Design review of the part built by this model. Coordinates are the model's own, in mm. A direction names the side the tool comes from. Coordinates: 2 decimals unless noted, no trailing zeros. Write each loop counter-clockwise with the first axis right and the second up, starting at its lowest first coordinate (ties: lowest second). Pieces come first, ordered by that corner, then holes. Notation, with made-up numbers: (62, -3.5) -> (73, -3.5) arc R16 ccw to (73, 2.5) -> close; hole circle Ø8 at (89.5, 29). An arc over 180 degrees is marked (long way). One line per question, with ' | ' between items. Start each with the question number.
Q1. Add section B-B on z = -4. State the section outline as (x, y) points, and give its area (3 significant figures).
Q2. For P1, Ø2, axis at x = 3, z = 1.5, coming from the +Y side; P2, Ø1.8, axis at x = -0.5, y = 0.5, coming from the -Z side (3 decimals); P3, Ø1.5, axis at y = 1, z = 3, coming from the -X side; P4, Ø10, axis at y = 3, z = 7, coming from the +X side, all flat-tipped, find the tip position at first contact; note any pin that passes through.
Q3. Add section A-A on y = 7.5. State the section outline as (x, z) points.
Q4. Add section C-C on y = -6. State the section outline as (x, z) points.
Q5. Add section D-D on x = 0. State the section outline as (y, z) points (3 decimals), and give its area (3 significant figures).
Q6. For faces 1 (the flat face through (0, 0, 12.5)), 2 (the flat face through (-4.762, -1, -11)), 3 (the flat face through (5.08, 7, 0)), list the 3-axis set-ups (+Z, -Z, +X, -X, +Y, -Y) from which the entire face can be reached by the end or side of a thin tool; tool diameter is ignored.
Q7. Wall thickness on probe 1 along Y at (x, z) = (0, -1.25); probe 2 along X at (y, z) = (6, 8.5); probe 3 along X at (y, z) = (5.5, 10): over which ranges is each line inside the solid? List them lowest first.
Q8. Draft analysis for pull direction X (two halves, no side actions). For faces 4 (the cylindrical face through (20.5, -0.13, 11.47)), 5 (the flat face through (4.762, -1, -11)), 6 (the flat face through (11, 9.6, 3)), state which applies: pulls with the +X half, pulls with the -X half, needs draft (parallel to the pull), parting line crosses it, or undercut.
from build123d import *

# Parameters (mm, degrees)
BOSS_EXTRUDE1_DEPTH = 9.6
FILLET5_R           = 2
SKETCH7_W           = 10.16
SKETCH7_H           = 5.28
CUT_EXTRUDE6_DEPTH  = 34.879754173
SKETCH11_W          = 9.525
SKETCH11_H          = 9.525
CUT_EXTRUDE9_DEPTH  = 3.375
SKETCH12_R          = 1.5
CUT_EXTRUDE10_DEPTH = 9.525


with BuildPart() as part:
    # Sketch1 → Boss-Extrude1 (new, symmetric)
    with BuildSketch(Plane(origin=(0, 0, 0), x_dir=(1, 0, 0), z_dir=(0, 1, 0))):
        Polygon((-14.297771125, -12.5), (14.297771125, -12.5), (22.216878365, -12.5), (7.783121635, 12.5), (-7.783121635, 12.5), (-22.216878365, -12.5), align=None)
    extrude(amount=BOSS_EXTRUDE1_DEPTH, both=True)

    # Fillet5
    fillet5_edges = [part.edges().sort_by_distance(p)[0] for p in [
        (-22.216878365, 0, 12.5),
        (-7.783121635, 0, -12.5),
        (7.783121635, 0, -12.5),
        (22.216878365, 0, 12.5),
    ]]
    fillet(fillet5_edges, radius=FILLET5_R)

    # Sketch7 → Cut-Extrude6 (cut, through all)
    with BuildSketch(Plane.XY.offset(12.5)):
        with Locations((0, 6.96)):
            Rectangle(SKETCH7_W, SKETCH7_H)
    extrude(amount=-CUT_EXTRUDE6_DEPTH, mode=Mode.SUBTRACT)

    # Sketch11 → Cut-Extrude9 (cut)
    with BuildSketch(Plane(origin=(0, 0, -12.5), x_dir=(-1, 0, 0), z_dir=(0, 0, -1))):
        with Locations((0, -0.4425)):
            Rectangle(SKETCH11_W, SKETCH11_H)
    extrude(amount=-CUT_EXTRUDE9_DEPTH, mode=Mode.SUBTRACT)

    # Sketch12 → Cut-Extrude10 (cut)
    with BuildSketch(Plane(origin=(0, 4.32, 0), x_dir=(1, 0, 0), z_dir=(0, 1, 0))):
        with Locations((3.2625, 9.125)):
            Circle(SKETCH12_R)
        with Locations((-3.2625, 9.125)):
            Circle(SKETCH12_R)
    extrude(amount=-CUT_EXTRUDE10_DEPTH, mode=Mode.SUBTRACT)


solid = part.part
Output values:
1) outline: (-12.69, -9.6) -> (12.69, -9.6) -> (12.69, 9.6) -> (5.08, 9.6) -> (5.08, 4.32) -> (-5.08, 4.32) -> (-5.08, 9.6) -> (-12.69, 9.6) -> close | area: 434 mm2
2) P1: stops at y = 4.32 | P2: stops at z = -9.125 | P3: stops at x = -17.17 | P4: stops at x = 20.75
3) outline: (-20.48, 9.5) -> (-8.36, -11.5) arc R2 ccw to (-6.63, -12.5) -> (-5.08, -12.5) -> (-5.08, 12.5) -> (-18.75, 12.5) arc R2 ccw to start; (5.08, -12.5) -> (6.63, -12.5) arc R2 ccw to (8.36, -11.5) -> (20.48, 9.5) arc R2 ccw to (18.75, 12.5) -> (5.08, 12.5) -> close
4) outline: (-20.48, 9.5) -> (-8.36, -11.5) arc R2 ccw to (-6.63, -12.5) -> (6.63, -12.5) arc R2 ccw to (8.36, -11.5) -> (20.48, 9.5) arc R2 ccw to (18.75, 12.5) -> (-18.75, 12.5) arc R2 ccw to start
5) outline: (-9.6, -12.5) -> (-5.205, -12.5) -> (-5.205, -9.125) -> (4.32, -9.125) -> (4.32, 12.5) -> (-9.6, 12.5) -> close | area: 316 mm2
6) face 1: +Z, +X, -X, +Y, -Y | face 2: -Z, +Y | face 3: +Z, -Z, +Y
7) probe 1: y = -9.6 to 4.32 | probe 2: x = -19.91 to -5.08, 5.08 to 19.91 | probe 3: x = -20.69 to -5.08, 5.08 to 20.69
8) face 4: pulls with the +X half | face 5: undercut | face 6: needs draft
